from build123d import *

# Parameters (mm, degrees)
SKETCH_1_W      = 110
SKETCH_1_H      = 43
SKETCH_1_R      = 19
SKETCH_1_R_2    = 1.5
EXTRUDE_2_DEPTH = 5
SKETCH_2_W      = 5
SKETCH_2_H      = 43
EXTRUDE_4_DEPTH = 37


with BuildPart() as part:
    # 草图1 → 凸台-拉伸2 (new body)
    with BuildSketch(Plane.XY):
        with Locations((25.61465721, 4.254137116)):
            Rectangle(SKETCH_1_W, SKETCH_1_H)
        with Locations((58.61465721, 4.254137116)):
            Circle(SKETCH_1_R, mode=Mode.SUBTRACT)
        with Locations((74.61465721, 20.254137116)):
            Circle(SKETCH_1_R_2, mode=Mode.SUBTRACT)
        with Locations((74.61465721, -11.745862884)):
            Circle(SKETCH_1_R_2, mode=Mode.SUBTRACT)
        with Locations((42.61465721, -11.745862884)):
            Circle(SKETCH_1_R_2, mode=Mode.SUBTRACT)
        with Locations((42.61465721, 20.254137116)):
            Circle(SKETCH_1_R_2, mode=Mode.SUBTRACT)
        with Locations((34.61465721, -11.745862884)):
            Circle(SKETCH_1_R_2, mode=Mode.SUBTRACT)
        with Locations((2.61465721, -11.745862884)):
            Circle(SKETCH_1_R_2, mode=Mode.SUBTRACT)
        with Locations((2.61465721, 20.254137116)):
            Circle(SKETCH_1_R_2, mode=Mode.SUBTRACT)
        with Locations((34.61465721, 20.254137116)):
            Circle(SKETCH_1_R_2, mode=Mode.SUBTRACT)
        with Locations((18.61465721, 4.254137116)):
            Circle(SKETCH_1_R, mode=Mode.SUBTRACT)
    extrude(amount=EXTRUDE_2_DEPTH)

    # 草图2 → 凸台-拉伸4 (add)
    with BuildSketch(Plane.XY.offset(5)):
        with Locations((83.11465721, 4.254137116)):
            Rectangle(SKETCH_2_W, SKETCH_2_H)
        with Locations((-31.88534279, 4.254137116)):
            Rectangle(SKETCH_2_W, SKETCH_2_H)
    extrude(amount=-EXTRUDE_4_DEPTH)


solid = part.part
Model file for the job. Use its own axes, mm. A direction names the side the tool comes from. Round coordinates to 2 decimals unless told otherwise and drop trailing zeros. Loops run counter-clockwise (first coordinate to the right, second up) from the corner with the lowest first, then second, coordinate; pieces in that order, holes last. Notation, with made-up numbers: M 54.5,-10 L 87.5,-10 A28 cw 87.5,15 Z; hole C -40,30.5 d2. An arc over 180 degrees is marked long. One line per question, with ' | ' between items.
1) Band-saw the part on D-D (y = 0). Give the cut face in (x, z), then the cut area to 3 significant figures.
Solved:
outline: M -34.39,-32 L -29.39,-32 L -29.39,0 L 0.1,0 L 0.1,5 L -34.39,5 Z; M 37.13,0 L 40.1,0 L 40.1,5 L 37.13,5 Z; M 77.13,0 L 80.61,0 L 80.61,-32 L 85.61,-32 L 85.61,5 L 77.13,5 Z | area: 550 mm²
2) Drill centre lines: line 1 along X through (y, z) = (12.5, -6.5); line 2 along Z through (x, y) = (-16, 17); line 3 along Y through (x, z) = (44.5, 3) (3 decimals). Where is each one in solid material? Low to high.
Solved:
line 1: x = -34.39 to -29.39, 80.61 to 85.61 | line 2: z = 0 to 5 | line 3: y = -17.246 to -8.465, 16.973 to 25.754
3) Mould opens along X. For faces 1 (the flat face through (25.3, -17.246, 0.3)), 2 (the cylindrical face through (44.045, 20.705, 2.465)), 3 (the flat face through (-34.385, 4, -13)), 4 (the cylindrical face through (36.045, -11.295, 2.465)) say: +X half, -X half, draft (parallel to the pull), parting line (faces both ways), or undercut.
Solved:
face 1: draft | face 2: undercut | face 3: -X half | face 4: undercut
4) Band-saw the part on C-C (y = 13). Give the cut face in (x, z).
Solved:
outline: M -34.39,-32 L -29.39,-32 L -29.39,0 L 1.75,0 L 1.75,5 L -34.39,5 Z; M 35.48,0 L 41.75,0 L 41.75,5 L 35.48,5 Z; M 75.48,0 L 80.61,0 L 80.61,-32 L 85.61,-32 L 85.61,5 L 75.48,5 Z
5) 3-axis set-ups, long thin cutter, end or side, ignore diameter. For faces 5 (the flat face through (80.615, 4, -16)), 6 (the cylindrical face through (36.045, 20.705, 2.465)): which of +Z, -Z, +X, -X, +Y, -Y reach the whole face in a straight line?
Solved:
face 5: -Z, +Y, -Y | face 6: +Z, -Z
6) Flat gauge pin, fed straight in: pin 1 (21.5 mm diameter, centred on x = 49.5, y = 11.5, fed in from -Z). Where does the tip first touch, or does it go through?
Solved:
pin 1: stops at z = 0
7) Band-saw the part on B-B (x = 29.5). Give the cut face in (y, z).
Solved:
outline: M -17.25,0 L -11.32,0 L -11.32,5 L -17.25,5 Z; M 19.83,0 L 25.75,0 L 25.75,5 L 19.83,5 Z
8) Band-saw the part on A-A (z = -3.5). Give the cut face in (x, y), then the cut area to 3 significant figures.
Solved:
outline: M -34.39,-17.25 L -29.39,-17.25 L -29.39,25.75 L -34.39,25.75 Z; M 80.61,-17.25 L 85.61,-17.25 L 85.61,25.75 L 80.61,25.75 Z | area: 430 mm²
